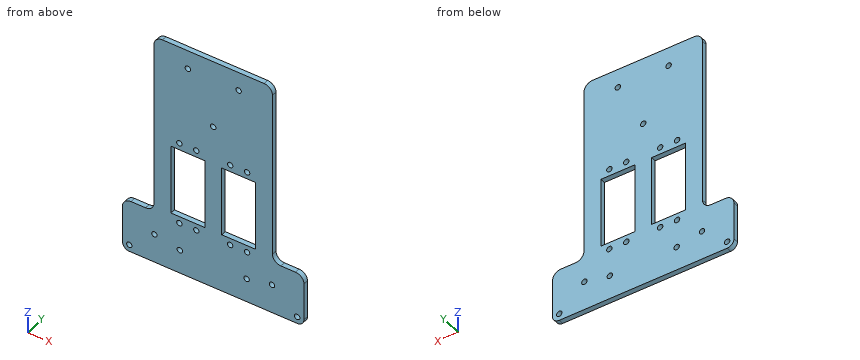
```python
from build123d import *

# Parameters (mm, degrees)
SKETCH013_R     = 1.6
SKETCH013_W     = 20
SKETCH013_H     = 41
PAD005_DEPTH    = 3
FILLET009_R     = 4
FILLET010_R     = 5
SKETCH019_R     = 1.6
POCKET011_DEPTH = 3.001


with BuildPart() as part:
    # Sketch013 (on DatumPlane) → Pad005 (new body)
    with BuildSketch(Plane.XZ.offset(41.112698)):
        Polygon((42.75, 129.5), (42.75, -9), (-10.85, -9), (-10.85, 22), (7.75, 22), (7.75, 129.5), align=None)
        with Locations((22.75, 21.5)):
            Circle(SKETCH013_R, mode=Mode.SUBTRACT)
        with Locations((32.75, 21.5)):
            Circle(SKETCH013_R, mode=Mode.SUBTRACT)
        with Locations((8, 8)):
            Circle(SKETCH013_R, mode=Mode.SUBTRACT)
        with Locations((-6.85, -5)):
            Circle(SKETCH013_R, mode=Mode.SUBTRACT)
        with Locations((23, 5)):
            Circle(SKETCH013_R, mode=Mode.SUBTRACT)
        with Locations((22.75, 70.5)):
            Circle(SKETCH013_R, mode=Mode.SUBTRACT)
        with Locations((32.75, 70.5)):
            Circle(SKETCH013_R, mode=Mode.SUBTRACT)
        with Locations((27.75, 46)):
            Rectangle(SKETCH013_W, SKETCH013_H, mode=Mode.SUBTRACT)
    pad005 = extrude(amount=PAD005_DEPTH)

    # Mirrored: Pad005 across face of Pad005
    add(pad005.mirror(Plane(origin=(42.75, -42.612698, 60.25), x_dir=(0, 1, 0), z_dir=(1, 0, 0))))

    # Fillet009
    fillet009_edges = [part.edges().sort_by_distance(p)[0] for p in [
        (96.35, -42.612698, -9),
        (-10.85, -42.612698, -9),
    ]]
    fillet(fillet009_edges, radius=FILLET009_R)

    # Fillet010
    fillet010_edges = [part.edges().sort_by_distance(p)[0] for p in [
        (77.75, -42.612698, 22),
        (96.35, -42.612698, 22),
        (-10.85, -42.612698, 22),
        (7.75, -42.612698, 22),
        (7.75, -42.612698, 129.5),
        (77.75, -42.612698, 129.5),
    ]]
    fillet(fillet010_edges, radius=FILLET010_R)

    # Sketch019 (on Face2 of Fillet010) → Pocket011 (cut, through all)
    with BuildSketch(Plane(origin=(0, -41.112698, 0), x_dir=(-1, 0, 0), z_dir=(0, 1, 0))):
        with Locations((-42.75, 89.5)):
            Circle(SKETCH019_R)
        with Locations((-57.75, 118.5)):
            Circle(SKETCH019_R)
        with Locations((-27.75, 118.5)):
            Circle(SKETCH019_R)
    extrude(amount=-POCKET011_DEPTH, mode=Mode.SUBTRACT)


solid = part.part
```
Geometry check sheet. Reference: the model listing, model coordinates, mm. Give positions to 0.01 mm unless a question says otherwise; leave off trailing zeros. Order: outer loops, then holes, each group sorted by start corner. A loop starts at its lowest first (then second) coordinate and runs counter-clockwise, first axis right, second up. Notation, with made-up numbers: (42.25, 20) - (85.25, 20) arc R13 cw to (85.25, 43) - close; hole circle Ø10 at (3.5, -26.5). An arc over 180 degrees is marked (long way). Answer in a Markdown table with one row per item. Add a question column.
Q1. Material ranges on probe 1 along Z at (x, y) = (27.75, -41.65); probe 2 along X at (y, z) = (-41.35, 28); probe 3 along Z at (x, y) = (22.75, -41.75), recorded low to high. Write a range as from..to.
Q2. Cross-section at A-A, the plane z = 34.5. Enter the section's corners in (x, y).
Q3. Cross-section at B-B, the plane x = 32.75. Enter the section's corners in (y, z), then the cut area to 3 significant figures.
Q4. Cross-section at C-C, the plane y = -43.3. Count the separate pieces of the cut face and the enclosed holes in it, then the cut area to 3 significant figures.
Q5. Gauge pin test, flat ends, axial feed: pin 1 (1.9 mm diameter, centred on x = 52.75, z = 70.5, fed in from +Y); pin 2 (1.5 mm diameter, centred on y = -42.5, z = 59, fed in from +X); pin 3 (0.9 mm diameter, centred on x = 86, y = -42.5, fed in from +Z). Record the tip position at first contact, or that the pin passes through.
Q6. Cross-section at D-D, the plane x = 0. Enter the section's corners in (y, z), then the cut area to 3 significant figures.
Check values:
| question | item | result |
|---|---|---|
| 1 | probe 1 | z = -9..25.5, 66.5..116.9, 120.1..129.5 |
| 1 | probe 2 | x = 7.75..17.75, 37.75..47.75, 67.75..77.75 |
| 1 | probe 3 | z = -9..3.42, 6.58..19.9, 23.1..25.5, 66.5..68.9, 72.1..129.5 |
| 2 | outline | (7.75, -44.11) - (17.75, -44.11) - (17.75, -41.11) - (7.75, -41.11) - close; (37.75, -44.11) - (47.75, -44.11) - (47.75, -41.11) - (37.75, -41.11) - close; (67.75, -44.11) - (77.75, -44.11) - (77.75, -41.11) - (67.75, -41.11) - close |
| 3 | outline | (-44.11, -9) - (-41.11, -9) - (-41.11, 19.9) - (-44.11, 19.9) - close; (-44.11, 23.1) - (-41.11, 23.1) - (-41.11, 25.5) - (-44.11, 25.5) - close; (-44.11, 66.5) - (-41.11, 66.5) - (-41.11, 68.9) - (-44.11, 68.9) - close; (-44.11, 72.1) - (-41.11, 72.1) - (-41.11, 129.5) - (-44.11, 129.5) - close |
| 3 | area | 273 mm^2 |
| 4 | separate pieces | 1 |
| 4 | enclosed holes | 19 |
| 4 | area | 9,050 mm^2 |
| 5 | pin 1 | passes through |
| 5 | pin 2 | stops at x = 77.75 |
| 5 | pin 3 | stops at z = 22 |
| 6 | outline | (-44.11, -9) - (-41.11, -9) - (-41.11, 22) - (-44.11, 22) - close |
| 6 | area | 93.0 mm^2 |
